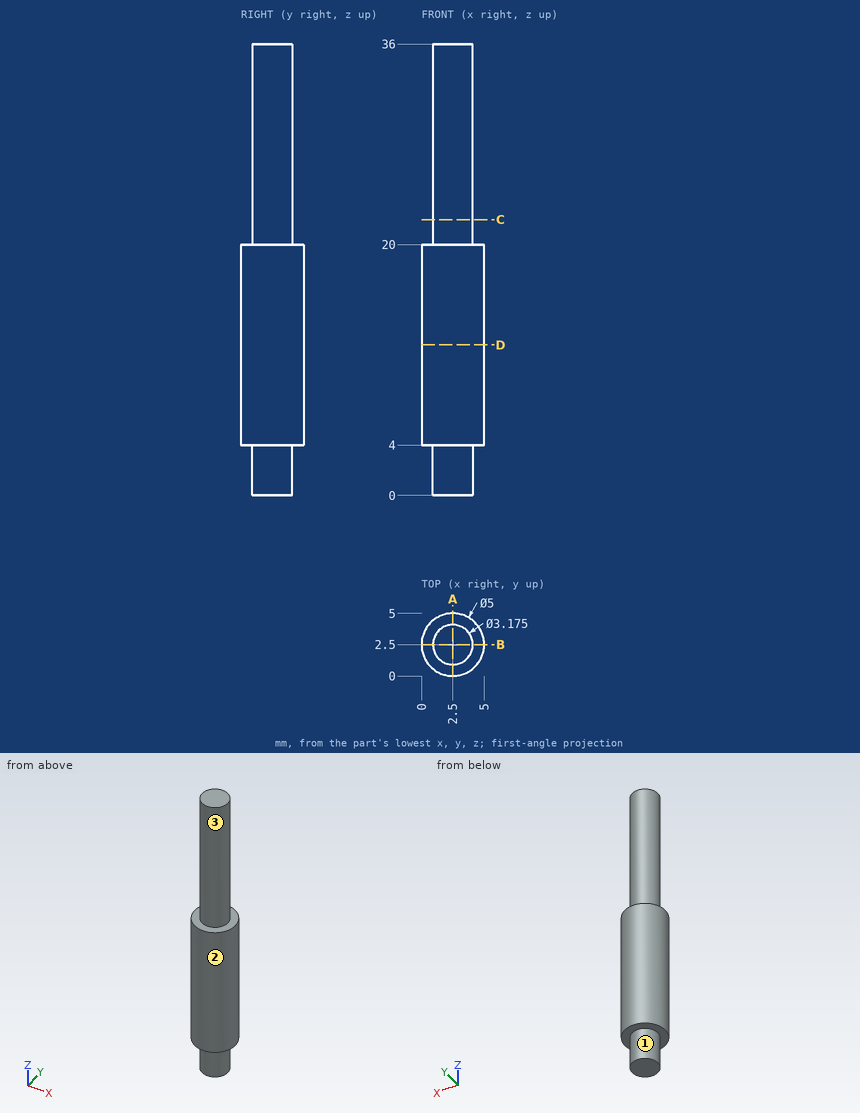
Can you work these out from the drawing? Everything is in mm from the part's minimum corner. A direction names the side the tool comes from. Give positions to 0.01 mm unless a question says otherwise; leave off trailing zeros. Loops run counter-clockwise (first coordinate to the right, second up) from the corner with the lowest first, then second, coordinate; pieces in that order, holes last. Notation, with made-up numbers: M -16.75,62 L 33.25,62 A18 ccw 33.25,95 Z; hole C 72,75 d1. An arc over 180 degrees is marked long. Put each result on its own line as item: value. Start each with the question number.
(1) I want a section at D-D on z = 12. Please give me the cut outline in (x, y).
(2) I want a section at A-A on x = 2.5. Please give me the cut outline in (y, z).
(3) I need wall thicknesses on line 1 along Z through (x, y) = (2.25, 0.85); line 2 along X through (y, z) = (2, 29); line 3 along X through (y, z) = (3.95, 12). Which ranges of each line are inside material? Lowest first, please. Write a range as [from, to].
(4) Will these pins go through, and if not, where does the flat tip stop? pin 1 Ø2 at (x, z) = (1, 15) entering from -Y; pin 2 Ø1.5 at (x, y) = (4, 0.5) entering from +Z.
(5) I want a section at C-C on z = 22. Please give me the cut outline in (x, y) (1 decimal), then the cut area to 3 significant figures.
(6) For the marked faces 1, 2 and 3, which set-ups out of +Z, -Z, +X, -X, +Y, -Y let a thin tool reach every point of the face, with its end or its side?
Answer block:
1. outline: C 2.5,2.5 d5
2. outline: M 0,4 L 0.91,4 L 0.91,0 L 4.09,0 L 4.09,4 L 5,4 L 5,20 L 4.09,20 L 4.09,36 L 0.91,36 L 0.91,20 L 0,20 Z
3. line 1: [4, 20]
3. line 2: [0.99, 4.01]
3. line 3: [0.46, 4.54]
4. pin 1: y = 0.05
4. pin 2: z = 20
5. outline: C 2.5,2.5 d3.2
5. area: 7.92 mm^2
6. face 1: -Z
6. face 2: +Z, -Z
6. face 3: +Z
